CAD build for the part. Positions are in the model's coordinates, mm. A direction names the side the tool comes from. Give positions to 0.01 mm unless a question says otherwise; leave off trailing zeros. Write each loop counter-clockwise with the first axis right and the second up, starting at its lowest first coordinate (ties: lowest second). Pieces come first, ordered by that corner, then holes. Notation, with made-up numbers: (-12, -15.75) -> (40, -15.75) arc R23 cw to (40, 2.25) -> close; hole circle Ø11 at (1, 6). An arc over 180 degrees is marked (long way). Answer as a JSON object with one key per item and string values.
```python
from build123d import *

# Parameters (mm, degrees)
F1_DEPTH = 34


with BuildPart() as f1:
    # F0 (on Right) → F1 (new body)
    with BuildSketch(Plane.YZ):
        with BuildLine():
            ThreePointArc((-26.890983, 1800.32203), (-43.892365, 1811.317181), (-64.131767, 1811.871154))
            Line((-64.131767, 1811.871154), (-90.982187, 1803.963156))
            ThreePointArc((-90.982187, 1803.963156), (-95.864249, 1800.742189), (-98.109715, 1795.341538))
            Line((-98.109715, 1795.341538), (-99.371331, 1782.409853))
            ThreePointArc((-99.371331, 1782.409853), (-99.138499, 1779.088701), (-97.828286, 1776.028048))
            Line((-97.828286, 1776.028048), (-94.050036, 1770.155742))
            ThreePointArc((-94.050036, 1770.155742), (-92.865546, 1767.564766), (-92.459738, 1764.744928))
            Line((-92.459738, 1764.744928), (-92.459738, 1750.292804))
            ThreePointArc((-92.459738, 1750.292804), (-87.867403, 1745.703047), (-83, 1750))
            Line((-83, 1750), (-80.388879, 1777.877985))
            ThreePointArc((-80.388879, 1777.877985), (-56.279235, 1800.967893), (-29.977198, 1780.41013))
            Line((-29.977198, 1780.41013), (-28.255004, 1750))
            Line((-28.255004, 1750), (-25.470103, 1750))
            Line((-25.470103, 1750), (-25.470103, 1686.175056))
            Line((-25.470103, 1686.175056), (28.529897, 1686.175056))
            Line((28.529897, 1686.175056), (28.529897, 1751.175056))
            Line((28.529897, 1751.175056), (22.537481, 1754.025714))
            ThreePointArc((22.537481, 1754.025714), (17.84148, 1756.482182), (13.345133, 1759.28745))
            Line((13.345133, 1759.28745), (-26.890983, 1800.32203))
        make_face()
    extrude(amount=F1_DEPTH)


solid = f1.part
```
1) Slice it at A-A (x = 20.5). List the corners of the cut face in (y, z) (3 decimals), then the cut area to 3 significant figures.
Model answer:
{"outline": "(-99.371, 1782.41) arc R10 ccw to (-97.828, 1776.028) -> (-94.05, 1770.156) arc R10 cw to (-92.46, 1764.745) -> (-92.46, 1750.293) arc R4.741 ccw to (-83, 1750) -> (-80.389, 1777.878) arc R25.5 cw to (-29.977, 1780.41) -> (-28.255, 1750) -> (-25.47, 1750) -> (-25.47, 1686.175) -> (28.53, 1686.175) -> (28.53, 1751.175) -> (22.537, 1754.026) arc R69.885 cw to (13.345, 1759.287) -> (-26.891, 1800.322) arc R37.5 ccw to (-64.132, 1811.871) -> (-90.982, 1803.963) arc R10 ccw to (-98.11, 1795.342) -> close", "area": "6,430 mm2"}
2) 3-axis set-ups, long thin cutter, end or side, ignore diameter. For faces 1 (the flat face through (17, -92.46, 1758)), 2 (the flat face through (17, -27, 1750)), 3 (the flat face through (16.762, -6.491, 1779.517)): which of +Z, -Z, +X, -X, +Y, -Y reach the whole face in a straight line?
Model answer:
{"face 1": "-Z, +X, -X, -Y", "face 2": "-Z, +X, -X", "face 3": "+Z, +X, -X, +Y"}
3) Slice it at C-C (z = 1788.5). List the corners of the cut face in (x, y).
Model answer:
{"outline": "(0, -98.78) -> (34, -98.78) -> (34, -76.94) -> (0, -76.94) -> close; (0, -33.06) -> (34, -33.06) -> (34, -15.3) -> (0, -15.3) -> close"}
4) Mould opens along Y. For faces 4 (the flat face through (16.76, -29.13, 1765.42)), 5 (the flat face through (16.76, 25.58, 1752.58)), 6 (the cylindrical face through (16.76, -43.62, 1811.23)) say: released by +Y, released by -Y, zero draft, split by the parting line, or undercut.
Model answer:
{"face 4": "undercut", "face 5": "released by +Y", "face 6": "split by the parting line"}
5) Wall check: probe 1 along Y at (x, z) = (18.5, 1707.5); probe 2 along Y at (x, z) = (8, 1768); probe 3 along Z at (x, y) = (23, -54). Give the ranges that are in metal, low to high.
Model answer:
{"probe 1": "y = -25.47 to 28.53", "probe 2": "y = -93 to -81.31, -29.27 to 4.8", "probe 3": "z = 1800.98 to 1812.99"}
6) Pin check, flat tips, straight feed: pin 1 (0.8 mm diameter, centred on x = 14.5, y = -26.5, fed in from -Z); pin 2 (7 mm diameter, centred on x = 19.5, z = 1757, fed in from -Y); pin 3 (1 mm diameter, centred on x = 22.5, z = 1792.5, fed in from -Y). Stop position of each tip, or through.
Model answer:
{"pin 1": "stops at z = 1750", "pin 2": "stops at y = -92.46", "pin 3": "stops at y = -98.44"}
7) Slice it at B-B (z = 1757.5). List the corners of the cut face in (x, y).
Model answer:
{"outline": "(0, -92.46) -> (34, -92.46) -> (34, -82.3) -> (0, -82.3) -> close; (0, -28.68) -> (34, -28.68) -> (34, 16.12) -> (0, 16.12) -> close"}
8) Slice it at D-D (y = -11). List the corners of the cut face in (x, z), then the cut area to 3 significant figures.
Model answer:
{"outline": "(0, 1686.18) -> (34, 1686.18) -> (34, 1784.12) -> (0, 1784.12) -> close", "area": "3,330 mm2"}
